Input: part model. Units: mm. Frame: model coordinates. Face numbers are marked on the shaded views. A direction names the side the tool comes from. Give positions to 0.01 mm unless a question says otherwise; leave off trailing zeros. Write each loop counter-clockwise with the first axis right and the second up, starting at its lowest first coordinate (ties: lowest second). Pieces come first, ordered by that corner, then holes. Notation, with made-up numbers: (27.5, -26) -> (72.5, -26) arc R6 ccw to (72.5, -19) -> close; hole circle Ø8 at (-39.75, 17). An arc over 180 degrees is marked (long way). Answer as a JSON object with one key per item and string values. Group by question number.
from build123d import *

# Parameters (mm, degrees)
F_1_5MM_DOWEL_HOLE1_D     = 1.5
F_1_5MM_DOWEL_HOLE1_DEPTH = 10
F_1_5MM_DOWEL_HOLE1_TIP   = 0.450645464
SKETCH3_R                 = 6
BOSS_EXTRUDE1_DEPTH       = 4.6
SKETCH7_R                 = 3
BOSS_EXTRUDE2_DEPTH       = 6
BOSS_EXTRUDE3_DEPTH       = 12


with BuildPart() as part:
    # Sketch2 one side → Revolve1 (revolve)
    with BuildSketch(Plane.XY, mode=Mode.PRIVATE) as revolve1_sk:
        Polygon((0, 37), (0, 18.5), (50, 18.5), (50, 23), (47, 23), (47, 34.9), (24, 34.9), (24, 37), align=None)
    revolve(revolve1_sk.sketch.rotate(Axis((0, 18.5, 0), (1, 0, 0)), 90), axis=Axis((0, 18.5, 0), (1, 0, 0)))

    # Sketch2_3 one side → Revolve2 (revolve)
    with BuildSketch(Plane.XY):
        Polygon((0, 37), (0, 18.5), (50, 18.5), (50, 23), (47, 23), (47, 34.9), (24, 34.9), (24, 37), align=None)
    revolve(axis=Axis((0, 18.5, 0), (1, 0, 0)))

    # 1.5mm Dowel Hole1
    with Locations(Plane.ZY):
        with Locations((-7.75, 31.923393759), (-15.5, 18.5), (-7.75, 5.076606241), (15.5, 18.5)):
            Hole(F_1_5MM_DOWEL_HOLE1_D / 2, depth=F_1_5MM_DOWEL_HOLE1_DEPTH)
            with Locations((0, 0, -(F_1_5MM_DOWEL_HOLE1_DEPTH + F_1_5MM_DOWEL_HOLE1_TIP / 2))):  # 118° drill point
                Cone(0, F_1_5MM_DOWEL_HOLE1_D / 2, F_1_5MM_DOWEL_HOLE1_TIP, mode=Mode.SUBTRACT)

    # Sketch3 → Boss-Extrude1 (add)
    with BuildSketch(Plane.ZY):
        with Locations((0, 11.5)):
            Circle(SKETCH3_R)
    extrude(amount=BOSS_EXTRUDE1_DEPTH)

    # Sketch7 → Boss-Extrude2 (add)
    with BuildSketch(Plane.ZY.offset(4.6)):
        with Locations((0, 11.5)):
            Circle(SKETCH7_R)
    extrude(amount=BOSS_EXTRUDE2_DEPTH)

    # Sketch8 → Boss-Extrude3 (add)
    with BuildSketch(Plane.ZY.offset(10.6)):
        with BuildLine():
            Line((-1.658312395, 14), (1.658312395, 14))
            ThreePointArc((1.658312395, 14), (0, 8.5), (-1.658312395, 14))
        make_face()
    extrude(amount=BOSS_EXTRUDE3_DEPTH)


solid = part.part
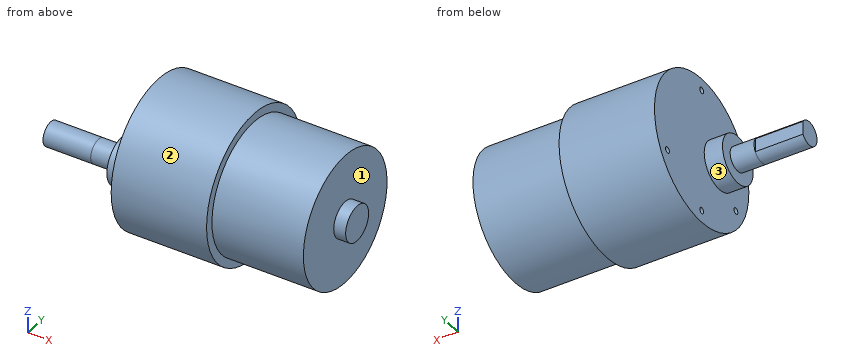
1. Section A-A (z = 0). Return the cut outline in (x, y), plus the area to 3 significant figures.
2. Section D-D (z = -12.5). Return the cut outline in (x, y).
3. Line query: line 1 (X direction, y = 9, z = 15); line 2 (X direction, y = 26, z = -9); line 3 (Y direction, x = 46.5, z = 0). Output: solid intervals per line, ascending.
4. Section B-B (y = 11.5). Return the cut outline in (x, z), plus the area to 3 significant figures.
5. Section C-C (x = 40). Return the cut outline in (y, z), plus the area to 3 significant figures.
6. Contact query for flat-ended pins moving along their axis: pin 1 Ø2 at (y, z) = (18.5, 15.5) entering from +X; pin 2 Ø1.5 at (x, y) = (-3, 15.5) entering from +Z; pin 3 Ø0.9 at (y, z) = (5.08, -7.75) entering from -X. Output: stop coordinate, or through.
7. Reachability of the marked faces 1, 2 and 3 from +Z, -Z, +X, -X, +Y, -Y: full face, straight path, thin tool, end or side. Return the list, or none.
Working result:
{
 "1": {"outline": "(-22.6, 8.5) -> (-4.6, 8.5) -> (-4.6, 5.5) -> (0, 5.5) -> (0, 0) -> (24, 0) -> (24, 2.1) -> (47, 2.1) -> (47, 14) -> (50, 14) -> (50, 23) -> (47, 23) -> (47, 34.9) -> (24, 34.9) -> (24, 37) -> (0, 37) -> (0, 17.5) -> (-4.6, 17.5) -> (-4.6, 14.5) -> (-10.6, 14.5) -> (-10.6, 14) -> (-22.6, 14) -> close", "area": "1,830 mm^2"},
 "2": {"outline": "(0, 4.86) -> (24, 4.86) -> (24, 7.88) -> (47, 7.88) -> (47, 29.12) -> (24, 29.12) -> (24, 32.14) -> (0, 32.14) -> close"},
 "3": {"line 1": "x = 0 to 24", "line 2": "x = 0 to 47", "line 3": "y = 2.1 to 34.9"},
 "4": {"outline": "(-22.6, -3) -> (-4.6, -3) -> (-4.6, -6) -> (0, -6) -> (0, -17.12) -> (24, -17.12) -> (24, -14.83) -> (47, -14.83) -> (47, 14.83) -> (24, 14.83) -> (24, 17.12) -> (0, 17.12) -> (0, 6) -> (-4.6, 6) -> (-4.6, 3) -> (-22.6, 3) -> close", "area": "1,670 mm^2"},
 "5": {"outline": "circle Ø32.8 at (18.5, 0)", "area": "845 mm^2"},
 "6": {"pin 1": "stops at x = 47", "pin 2": "stops at z = 5.04", "pin 3": "stops at x = 10.18"},
 "7": {"face 1": "+X", "face 2": "+X, -X", "face 3": "-X"}
}
